Check sheet for the modelled part. Datum: model origin and axes. Units: mm. A direction names the side the tool comes from. Give positions to 0.01 mm unless a question says otherwise; leave off trailing zeros. Order: outer loops, then holes, each group sorted by start corner. A loop starts at its lowest first (then second) coordinate and runs counter-clockwise, first axis right, second up.
Item 1: Sectioned sample at C-C on z = 104.5. Record the boundary of the cut face in (x, y).
Item 2: Material ranges on line 1 along Z through (x, y) = (-2.25, -5.75); line 2 along Y through (x, z) = (-5, 26); line 3 along Y through (x, z) = (-3, 41), recorded low to high.
Item 3: Sectioned sample at A-A on z = 75.5. Record the boundary of the cut face in (x, y), and give its area (3 significant figures).
Item 4: Access from +Z, -Z, +X, -X, +Y, -Y to the whole of each face (thin tool, end or side, straight path). Record for faces 1 (the flat face through (1, 3, 98)), 2 (the flat face through (2, 2, -5)), 3 (the cylindrical face through (3, 0, -3)).
Item 5: Release check for a two-part mould opening along Z. For faces 4 (the cylindrical face through (-7.493, 0.33, 47.821)), 5 (the flat face through (0, 0, 121)), 6 (the flat face through (0, 0, -11)), 7 (the cylindrical face through (0.54, -2.44, -5.35)) record: released by +Z, released by -Z, zero draft, split by the parting line, or undercut.
Item 6: Sectioned sample at B-B on x = 6. Record the boundary of the cut face in (y, z).
Item 7: Gauge pin test, flat ends, axial feed: P1, Ø2, axis at y = -5.5, z = 97, coming from the +X side; P2, Ø2, axis at x = 4, z = 15.5, coming from the +Y side; P3, Ø5, axis at y = -3, z = 32, coming from the -X side; P4, Ø5, axis at x = 3, y = 2, coming from the -Z side. Record the tip position at first contact, or that the pin passes through.
from build123d import *

# Parameters (mm, degrees)
SKETCH_1_R          = 7.5
EXTRUDE_1_DEPTH     = 97
SKETCH_2_R          = 4
EXTRUDE_2_DEPTH     = 1
SKETCH_3_R          = 3
EXTRUDE_3_DEPTH     = 10
SKETCH_4_R          = 4
EXTRUDE_4_DEPTH     = 1
SKETCH_5_R          = 3
EXTRUDE_5_DEPTH     = 23
SKETCH_6_R          = 6.147127497
SKETCH_6_R_2        = 2.5
CUT_EXTRUDE_1_DEPTH = 0.7
SKETCH_7_R          = 6.101942299
SKETCH_7_R_2        = 2.5
CUT_EXTRUDE_2_DEPTH = 0.7


with BuildPart() as part:
    # 草图1 → 凸台-拉伸1 (new body)
    with BuildSketch(Plane.XY):
        Circle(SKETCH_1_R)
    extrude(amount=EXTRUDE_1_DEPTH)

    # 草图2 → 凸台-拉伸2 (add)
    with BuildSketch(Plane(origin=(0, 0, 0), x_dir=(-1, 0, 0), z_dir=(0, 0, -1))):
        Circle(SKETCH_2_R)
    extrude(amount=EXTRUDE_2_DEPTH)

    # 草图3 → 凸台-拉伸3 (add)
    with BuildSketch(Plane(origin=(0, 0, -1), x_dir=(-1, 0, 0), z_dir=(0, 0, -1))):
        Circle(SKETCH_3_R)
    extrude(amount=EXTRUDE_3_DEPTH)

    # 草图4 → 凸台-拉伸4 (add)
    with BuildSketch(Plane.XY.offset(97)):
        Circle(SKETCH_4_R)
    extrude(amount=EXTRUDE_4_DEPTH)

    # 草图5 → 凸台-拉伸5 (add)
    with BuildSketch(Plane.XY.offset(98)):
        Circle(SKETCH_5_R)
    extrude(amount=EXTRUDE_5_DEPTH)

    # 草图6 → 切除-拉伸1 (cut)
    with BuildSketch(Plane(origin=(0, 0, -5), x_dir=(-1, 0, 0), z_dir=(0, 0, -1))):
        Circle(SKETCH_6_R)
        Circle(SKETCH_6_R_2, mode=Mode.SUBTRACT)
    extrude(amount=CUT_EXTRUDE_1_DEPTH, mode=Mode.SUBTRACT)

    # 草图7 → 切除-拉伸2 (cut)
    with BuildSketch(Plane(origin=(0, 0, 102), x_dir=(-1, 0, 0), z_dir=(0, 0, -1))):
        Circle(SKETCH_7_R)
        Circle(SKETCH_7_R_2, mode=Mode.SUBTRACT)
    extrude(amount=-CUT_EXTRUDE_2_DEPTH, mode=Mode.SUBTRACT)


solid = part.part
Report:
1. outline: circle Ø6 at (0, 0)
2. line 1: z = 0 to 97
2. line 2: y = -5.59 to 5.59
2. line 3: y = -6.87 to 6.87
3. outline: circle Ø15 at (0, 0)
3. area: 177 mm2
4. face 1: +Z
4. face 2: none
4. face 3: -Z
5. face 4: zero draft
5. face 5: released by +Z
5. face 6: released by -Z
5. face 7: undercut
6. outline: (-4.5, 0) - (4.5, 0) - (4.5, 97) - (-4.5, 97) - close
7. P1: stops at x = 6
7. P2: stops at y = 6.87
7. P3: stops at x = -7.48
7. P4: stops at z = -11
